Could you check a few things on this model? Use its own coordinates, in mm. A direction names the side the tool comes from. Give positions to 0.01 mm unless a question says otherwise; leave off trailing zeros. Write each loop counter-clockwise with the first axis right and the second up, starting at its lowest first coordinate (ties: lowest second). Pieces come first, ordered by that corner, then holes. Notation, with made-up numbers: (56, -15) - (71, -15) arc R10 ccw to (71, -6) - close; hole circle Ø4 at (44.5, -39.75). An arc over 180 degrees is marked (long way). Answer in a Markdown table with one row per item.
Autodesk Inventor part; units mm, degrees
ref_plane "YZ Plane" through (0, 0, 0) normal (1, 0, 0) x (0, 1, 0)
ref_plane "XZ Plane" through (0, 0, 0) normal (0, 1, 0) x (-1, 0, 0)
ref_plane "XY Plane" through (0, 0, 0) normal (0, 0, 1) x (1, 0, 0)
sketch "Sketch1" plane through (0, 0, 0) normal (0, 1, 0) x (-1, 0, 0)
  line L0 (-132.5, 287.3805) -> (-122.5, 287.3805)
  line L1 (-132.5, 20) -> (-132.5, 287.3805)
  line L2 (-122.5, 20) -> (-122.5, 287.3805)
  line L3 (77.5, 287.3805) -> (87.5, 287.3805)
  line L4 (77.5, 20) -> (77.5, 287.3805)
  line L5 (87.5, 20) -> (87.5, 287.3805)
  line L6 (82.5, 0) -> (127.5, 0) construction
  line L7 (-132.5, 20) -> (-132.5, 287.3805)
  line L8 (82.5, 45) -> (-127.5, 45)
  line L9 (82.5, 155) -> (-127.5, 155)
  circle A0 centre (-127.5, 265) radius 1.6
  circle A1 centre (-127.5, 155) radius 1.6
  circle A2 centre (-127.5, 45) radius 1.6
  circle A3 centre (82.5, 45) radius 1.6
  circle A4 centre (82.5, 155) radius 1.6
  circle A5 centre (82.5, 265) radius 1.6
  line L10 (-132.5, 287.3805) -> (87.5, 287.3805)
  line L11 (87.5, 287.3805) -> (87.5, 0)
  line L12 (87.5, 0) -> (-132.5, 0)
  line L13 (-132.5, 0) -> (-132.5, 287.3805)
  line L14 (87.5, 0) -> (-132.5, 0)
  line L15 (-132.5, 0) -> (-132.5, -22.8)
  line L16 (-132.5, -22.8) -> (87.5, -22.8)
  line L17 (87.5, -22.8) -> (87.5, 0)
  arc A6 (6, 100) -> (0, 94) centre (6, 94) ccw
  line L18 (0, 0) -> (0, 94)
  line L19 (0, 0) -> (90, 0)
  line L20 (90, 0) -> (90, 94)
  arc A7 (90, 94) -> (84, 100) centre (84, 94) ccw
  line L21 (6, 100) -> (84, 100)
  circle A8 centre (45, 47.3805) radius 11
  circle A9 centre (76.75, 79.1305) radius 5.75
  circle A10 centre (13.25, 15.6305) radius 5.75
  circle A11 centre (76.75, 15.6305) radius 5.75
  circle A12 centre (13.25, 79.1305) radius 5.75
  circle A13 centre (117.5, 135) radius 1.8
  line L22 (112.5, 267.3805) -> (122.5, 267.3805)
  line L23 (112.5, 0) -> (112.5, 267.3805)
  line L24 (112.5, 0) -> (122.5, 0)
  line L25 (122.5, 0) -> (122.5, 267.3805)
  circle A14 centre (117.5, 25) radius 1.8
  circle A15 centre (117.5, 245) radius 1.8
  circle A16 centre (-92.5, 135) radius 1.8
  line L26 (-97.5, 267.3805) -> (-87.5, 267.3805)
  line L27 (-97.5, 0) -> (-97.5, 267.3805)
  line L28 (-97.5, 0) -> (-87.5, 0)
  line L29 (-87.5, 0) -> (-87.5, 267.3805)
  circle A17 centre (-92.5, 245) radius 1.8
  circle A18 centre (-92.5, 25) radius 1.8
  point P0 (-62.5, 0)
  point P1 (52.5, -20)
  dimension "d0" = 45
  dimension "d2" = 110
  dimension "d4" = 3.2
  dimension "d5" = 3.2
  dimension "d6" = 3.2
  dimension "d7" = 3.2
  dimension "d8" = 3.2
  dimension "d9" = 3.2
  dimension "d12" = 22.8
extrude "Extrusion1" add sketch "Sketch1" along normal blind 3 contours L0 L2 L8 L27 L12 L13 L1 | L10 L4 L9 L29 L26 L27 L2 | L9 L27 L8 L2 | L3 L5 A7 L21 L4 | L27 L26 L29 L9 | L9 L29 L8 L27 | L4 L21 A6 L18 L8 L29 L9 | L27 L8 L29 L12 | L5 L11 L12 L18 L8 A8 L4 A9 L21 A7 | L4 A9 L8 A8 L18 A6 L21 | L29 L8 L18 L12 | A9 L4 | L4 A9 | A8 L8 | L8 A8 | A10 | A11 | A12 | A16 | A17 | A18
fillet "Fillet1" radius 20 2 edges at (132.5, 1.5, 0) (-87.5, 1.5, 0)
sketch "Sketch4" plane through (0, 0, 0) normal (0, -1, 0) x (1, 0, 0)
  line L0 (68.5, 205.2102) -> (31.5, 205.2102)
  line L1 (78.5, 192.2868) -> (21.5, 192.2868)
  line L2 (21.5, 205.2102) -> (31.5, 205.2102)
  line L3 (68.5, 205.2102) -> (78.5, 205.2102)
  line L4 (78.5, 205.2102) -> (78.5, 192.2868)
  line L5 (21.5, 192.2868) -> (21.5, 205.2102)
  circle A0 centre (21.75, 99.1305) radius 7.65
  circle A1 centre (-41.75, 99.1305) radius 7.65
  circle A2 centre (21.75, 35.6305) radius 7.65
  arc A3 (10, 67.3805) -> (-30, 67.3805) centre (-10, 67.3805) ccw
  line L6 (10, 67.3805) -> (10, -32.6195)
  line L7 (-30, -32.6195) -> (-30, 67.3805)
  circle A4 centre (-41.75, 35.6305) radius 7.65
  line L8 (-87.5, 20) -> (-87.5, 287.3805)
  line L9 (-87.5, 287.3805) -> (132.5, 287.3805)
  line L10 (132.5, 287.3805) -> (132.5, 20)
  line L11 (112.5, 0) -> (-67.5, 0)
  line L12 (-87.5, 20) -> (-87.5, 287.3805)
  line L13 (-87.5, 287.3805) -> (132.5, 287.3805)
  circle A5 centre (-41.75, 99.1305) radius 10
  circle A6 centre (21.75, 99.1305) radius 10
  circle A7 centre (-41.75, 35.6305) radius 10
  circle A8 centre (21.75, 35.6305) radius 10
  line L14 (-87.5, 287.3805) -> (132.5, 287.3805)
  line L15 (21.75, 287.3805) -> (78.5, 287.3805)
  line L16 (78.5, 287.3805) -> (78.5, 157.3805)
  line L17 (78.5, 157.3805) -> (21.75, 157.3805)
  line L18 (21.75, 157.3805) -> (21.75, 287.3805)
  circle A9 centre (-10, 67.3805) radius 13
  line L19 (80.125, 157.3805) -> (20.125, 157.3805)
  line L20 (20.125, 157.3805) -> (20.125, 287.3805)
  line L21 (20.125, 287.3805) -> (80.125, 287.3805)
  line L22 (80.125, 287.3805) -> (80.125, 157.3805)
  line L23 (80.125, 157.3805) -> (20.125, 287.3805) construction
  line L24 (20.125, 157.3805) -> (80.125, 287.3805) construction
  line L25 (-13.375, 287.3805) -> (113.625, 287.3805)
  line L26 (113.625, 287.3805) -> (113.625, 157.3805)
  line L27 (113.625, 157.3805) -> (-13.375, 157.3805)
  line L28 (-13.375, 157.3805) -> (-13.375, 287.3805)
  line L29 (-13.375, 287.3805) -> (113.625, 157.3805) construction
  line L30 (113.625, 287.3805) -> (-13.375, 157.3805) construction
  point P0 (0, 0)
  point P1 (50.125, 222.3805)
  dimension "d24" = 20
  dimension "d25" = 20
  dimension "d26" = 20
  dimension "d27" = 20
  dimension "d28" = 130
  dimension "d29" = 26
  dimension "d36" = 60
  dimension "d37" = 130
  dimension "d38" = 127
extrude "Extrusion3" cut sketch "Sketch4" against normal up to surface (3 mm away) contours L3 L4 L1 L18 L2 L0 | L0 L2 L18 L9 L16 L3 | L16 L9 L22 L19 L4 | L18 L1 L5 L2 | L2 L5 L1 L18 L19 L20 L9 | L16 L17 L18 L1 | L9 L26 L27 L22 | L20 L27 L28 L9 | A0 | A1 | A2 | A4 | A5 | A6 | A7 | A8 | A9
chamfer "Chamfer1" distance 10 angle 45 2 edges at (-13.375, 1.5, 287.3805) (113.625, 1.5, 287.3805)
sketch "Sketch5" plane through (0, 0, 0) normal (0, -1, 0) x (1, 0, 0)
  line L0 (113.625, 157.3805) -> (-13.375, 157.3805)
  line L1 (113.625, 157.3805) -> (93.625, 157.3805)
  line L2 (93.625, 157.3805) -> (93.625, 137.3805)
  line L3 (93.625, 137.3805) -> (80.325, 137.3805)
  line L4 (80.325, 137.3805) -> (80.325, 128.8805)
  line L5 (80.325, 128.8805) -> (93.625, 128.8805)
  line L6 (93.625, 128.8805) -> (93.625, 137.3805)
  line L7 (93.625, 133.1305) -> (100.625, 133.1305)
  circle A0 centre (100.625, 133.1305) radius 3
  line L8 (97.625, 133.1305) -> (97.625, 127.1305)
  line L9 (103.625, 133.1305) -> (103.625, 127.1305)
  line L10 (100.625, 133.1305) -> (100.625, 124.1305)
  circle A1 centre (100.625, 124.1305) radius 3
  line L11 (97.625, 127.1305) -> (97.625, 124.1305)
  line L12 (103.625, 127.1305) -> (103.625, 124.1305)
  point P0 (0, 0)
  dimension "d39" = 20
  dimension "d40" = 20
  dimension "d41" = 13.3
  dimension "d42" = 8.5
  dimension "d45" = 7
  dimension "d46" = 6
  dimension "d47" = 6
  dimension "d48" = 6
  dimension "d49" = 9
extrude "Extrusion4" cut sketch "Sketch5" against normal up to surface (3 mm away)
equation "\"BendRadius\" = Thickness"
equation "\"BendReliefWidth\" = Thickness"
equation "\"BendReliefDepth\" = 0.5 * Thickness"
equation "\"CornerReliefSize\" = 4 * Thickness"
equation "\"MinimumRemnant\" = 2 * Thickness"
equation "\"TransitionRadius\" = BendRadius"
equation "\"JacobiRadiusSize\" = Thickness"
equation "\"GapSize\" = Thickness"
properties part number "obudowa_zewnetrzna_tyl_korba" material "ABS Plastic"
1) If I drill on line 1 (X direction, y = 2.15, z = 155); line 2 (X direction, y = 1.25, z = 265) (3 decimals); line 3 (X direction, y = 0.75, z = 162) (3 decimals), over which ranges is the centre line in solid material (lowest first)?
Check values:
| item | result |
|---|---|
| line 1 | x = -87.5 to -84.1, -80.9 to 125.9, 129.1 to 132.5 |
| line 2 | x = -87.5 to -84.1, -80.9 to -13.375, 113.625 to 125.9, 129.1 to 132.5 |
| line 3 | x = -87.5 to -13.375, 113.625 to 132.5 |
2) Imagine slicing it at A-A (x = -41.75). List the corners of the cut face in (y, z) for me, then the cut area to 3 significant figures.
Check values:
| item | result |
|---|---|
| outline | (0, 0) - (3, 0) - (3, 25.63) - (0, 25.63) - close; (0, 45.63) - (3, 45.63) - (3, 89.13) - (0, 89.13) - close; (0, 109.13) - (3, 109.13) - (3, 287.38) - (0, 287.38) - close |
| area | 742 mm2 |
3) Imagine slicing it at D-D (y = 2.1). State how many separate pieces and enclosed holes the cut face has, then the cut area to 3 significant figures.
Check values:
| item | result |
|---|---|
| separate pieces | 1 |
| enclosed holes | 13 |
| area | 44,400 mm2 |
4) On a 3-axis mill with a long thin cutter (end or side, diameter ignored), from which of +Z, -Z, +X, -X, +Y, -Y can I reach the whole of each face in a straight line? I mean faces 5 (the face through (-81.486, 1.521, 5.703)), 6 (the face through (118.555, 1.479, 282.31)). Say none if no direction works.
Check values:
| item | result |
|---|---|
| face 5 | -Z, -X, +Y, -Y |
| face 6 | +Z, +Y, -Y |
5) We'd pull the mould along Z, two halves only. Please class faces 1 (the face through (24, 0, 114)), 2 (the face through (27.13, 1.48, 44.06)), 3 (the face through (-18.445, 1.479, 282.45)), 4 (the face through (-3.01, 1.48, 78.34)): +Z half, -Z half, draft (parallel to the pull), parting line (faces both ways), or undercut.
Check values:
| item | result |
|---|---|
| face 1 | draft |
| face 2 | undercut |
| face 3 | +Z half |
| face 4 | undercut |
6) Will these pins go through, and if not, where does the flat tip stop? P1, Ø1, axis at x = 30.5, y = 1.5, coming from the +Z side; P2, Ø8, axis at x = -61.5, z = 120, coming from the -Y side; P3, Ø12, axis at x = 21.75, z = 35.63, coming from the +Y side.
Check values:
| item | result |
|---|---|
| P1 | stops at z = 157.38 |
| P2 | stops at y = 0 |
| P3 | passes through |
7) Imagine slicing it at C-C (z = 195.5). List the corners of the cut face in (x, y) for me (3 decimals), then the cut area to 3 significant figures.
Check values:
| item | result |
|---|---|
| outline | (-87.5, 0) - (-13.375, 0) - (-13.375, 3) - (-87.5, 3) - close; (113.625, 0) - (132.5, 0) - (132.5, 3) - (113.625, 3) - close |
| area | 279 mm2 |
8) Imagine slicing it at B-B (x = -10). List the corners of the cut face in (y, z) for me, then the cut area to 3 significant figures.
Check values:
| item | result |
|---|---|
| outline | (0, 0) - (3, 0) - (3, 54.38) - (0, 54.38) - close; (0, 80.38) - (3, 80.38) - (3, 157.38) - (0, 157.38) - close |
| area | 394 mm2 |
